Can you work these out from the drawing? Everything is in mm from the part's minimum corner. A direction names the side the tool comes from. Round coordinates to 2 decimals unless told otherwise and drop trailing zeros. Loops run counter-clockwise (first coordinate to the right, second up) from the corner with the lowest first, then second, coordinate; pieces in that order, holes last. Notation, with made-up numbers: M -10,64 L 26,64 A18 cw 26,72 Z; hole C -36,75.25 d10. An arc over 180 degrees is marked long. Return JSON: item names as keys, results as strings. Group by question number.
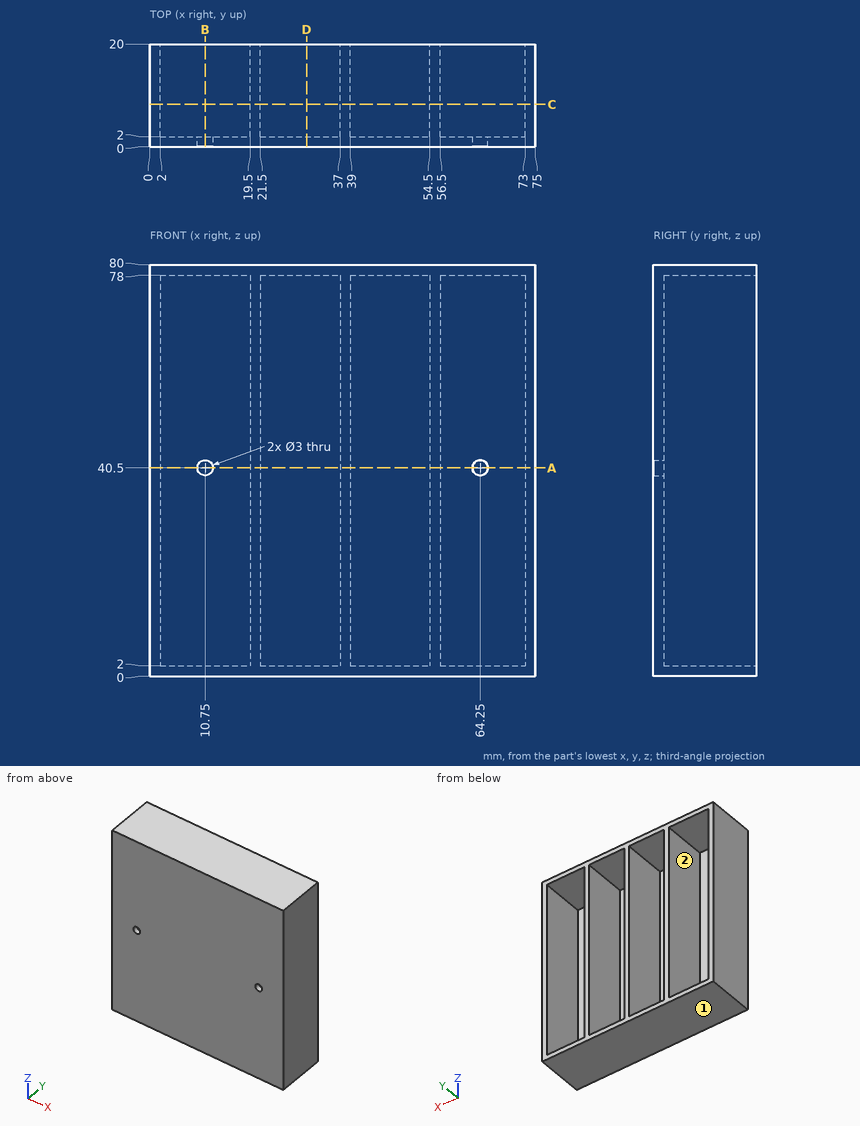
1. If we section it at B-B, the plane x = 10.75: Please give me the cut outline in (y, z), then the cut area to 3 significant figures.
2. If we section it at D-D, the plane x = 30.5: Please give me the cut outline in (y, z), then the cut area to 3 significant figures.
3. If we section it at A-A, the plane z = 40.5: Please give me the cut outline in (x, y).
4. I need wall thicknesses on probe 1 along X at (y, z) = (2.5, 67); probe 2 along X at (y, z) = (0.6, 40.5); probe 3 along Z at (x, y) = (58, 8.25). Which ranges of each line are inside material? Lowest first, please.
5. On a 3-axis mill with a long thin cutter (end or side, diameter ignored), from which of +Z, -Z, +X, -X, +Y, -Y can I reach the whole of each face in a straight line? I mean the marked faces 1 and 2. Say none if no direction works.
6. I'm going to push flat-ended pins straight in: pin 1 Ø3 at (y, z) = (6, 14.5) entering from -X; pin 2 Ø4.5 at (x, z) = (33, 35) entering from +Y; pin 3 Ø2.5 at (x, z) = (64.25, 40.5) entering from +Y. Where does each tip first touch, or does it pass through?
7. If we section it at C-C, the plane y = 8.25: Please give me the cut outline in (x, z).
Geometry results:
{
 "1": {"outline": "M 0,0 L 20,0 L 20,2 L 2,2 L 2,39 L 0,39 Z; M 0,42 L 2,42 L 2,78 L 20,78 L 20,80 L 0,80 Z", "area": "226 mm^2"},
 "2": {"outline": "M 0,0 L 20,0 L 20,2 L 2,2 L 2,78 L 20,78 L 20,80 L 0,80 Z", "area": "232 mm^2"},
 "3": {"outline": "M 0,0 L 9.25,0 L 9.25,2 L 2,2 L 2,20 L 0,20 Z; M 12.25,0 L 62.75,0 L 62.75,2 L 56.5,2 L 56.5,20 L 54.5,20 L 54.5,2 L 39,2 L 39,20 L 37,20 L 37,2 L 21.5,2 L 21.5,20 L 19.5,20 L 19.5,2 L 12.25,2 Z; M 65.75,0 L 75,0 L 75,20 L 73,20 L 73,2 L 65.75,2 Z"},
 "4": {"probe 1": "0 to 2, 19.5 to 21.5, 37 to 39, 54.5 to 56.5, 73 to 75", "probe 2": "0 to 9.25, 12.25 to 62.75, 65.75 to 75", "probe 3": "0 to 2, 78 to 80"},
 "5": {"face 1": "-Z, +X, -X, +Y, -Y", "face 2": "+Y"},
 "6": {"pin 1": "x = 0", "pin 2": "y = 2", "pin 3": "through"},
 "7": {"outline": "M 0,0 L 75,0 L 75,80 L 0,80 Z; hole M 2,2 L 19.5,2 L 19.5,78 L 2,78 Z; hole M 21.5,2 L 37,2 L 37,78 L 21.5,78 Z; hole M 39,2 L 54.5,2 L 54.5,78 L 39,78 Z; hole M 56.5,2 L 73,2 L 73,78 L 56.5,78 Z"}
}
